Answer from the drawing. Dimensions are ordinates in mm from the lowest x, y and z of the part. A direction names the side the tool comes from. Round coordinates to 2 decimals unless told otherwise and drop trailing zeros. Loops run counter-clockwise (first coordinate to the right, second up) from the corner with the lowest first, then second, coordinate; pieces in that order, holes last. Notation, with made-up numbers: (89.25, 16.5) - (102.25, 16.5) arc R29 cw to (102.25, 40.5) - close; hole circle Ø5 at (12.5, -11). An arc over 180 degrees is marked (long way). Use CSV: the item, a comma, the result in double quotes. Start each with the question number.
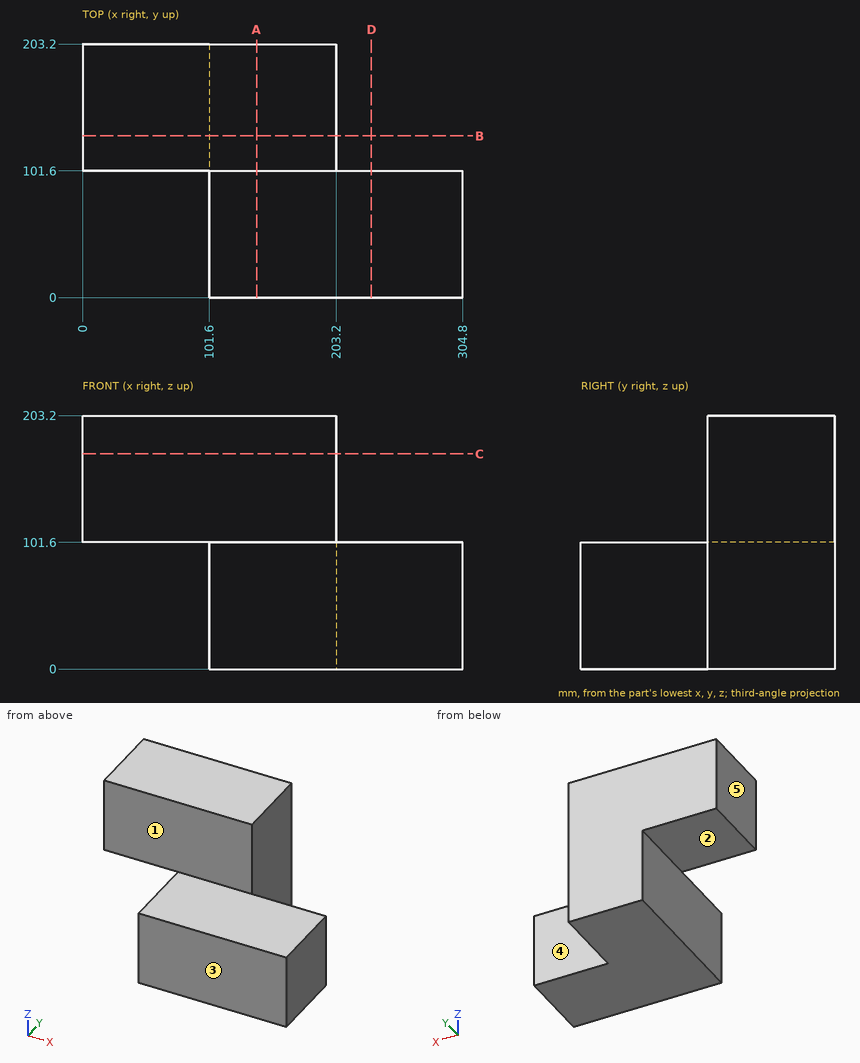
Item 1: A cutting plane is placed at D-D (x = 231.5). Determine the outline of the cut face in (y, z).
Item 2: Find the intervals of material crossed by probe 1 along Z at (x, y) = (290.5, 98); probe 2 along Y at (x, z) = (29, 147), in increasing order. Write a range as [from, to].
Item 3: A cutting plane is placed at B-B (y = 129.5). Determine the outline of the cut face in (x, z), plus the area to 3 significant figures.
Item 4: Each of these flat-tipped pins is pushed along its axis until it touches: pin 1 Ø6 at (x, y) = (204.5, 128.5) entering from -Z; pin 2 Ø6 at (x, y) = (249.5, 76.5) entering from +Z; pin 3 Ø10 at (y, z) = (141, 34) entering from -X; pin 4 Ø10 at (y, z) = (131, 162.5) entering from +X. Where does it stop, or does it pass through?
Item 5: A cutting plane is placed at C-C (z = 172.5). Determine the outline of the cut face in (x, y).
Item 6: Which of the six approach directions +Z, -Z, +X, -X, +Y, -Y give full straight-line access (tool end or side, diameter ignored) to the marked faces 1, 2, 3, 4 and 5?
Item 7: A cutting plane is placed at A-A (x = 139.5). Determine the outline of the cut face in (y, z), plus the area to 3 significant figures.
Result sheet:
1,outline,"(0, 0) - (101.6, 0) - (101.6, 101.6) - (0, 101.6) - close"
2,probe 1,"[0, 101.6]"
2,probe 2,"[101.6, 203.2]"
3,outline,"(0, 101.6) - (101.6, 101.6) - (101.6, 0) - (203.2, 0) - (203.2, 203.2) - (0, 203.2) - close"
3,area,"31,000 mm^2"
4,pin 1,"z = 0"
4,pin 2,"z = 101.6"
4,pin 3,"x = 101.6"
4,pin 4,"x = 203.2"
5,outline,"(0, 101.6) - (203.2, 101.6) - (203.2, 203.2) - (0, 203.2) - close"
6,face 1,"+Z, +X, -X, -Y"
6,face 2,"-Z, -X, +Y, -Y"
6,face 3,"+Z, -Z, +X, -X, -Y"
6,face 4,"+Z, -Z, +X, +Y"
6,face 5,"+Z, -Z, -X, +Y, -Y"
7,outline,"(0, 0) - (203.2, 0) - (203.2, 203.2) - (101.6, 203.2) - (101.6, 101.6) - (0, 101.6) - close"
7,area,"31,000 mm^2"
